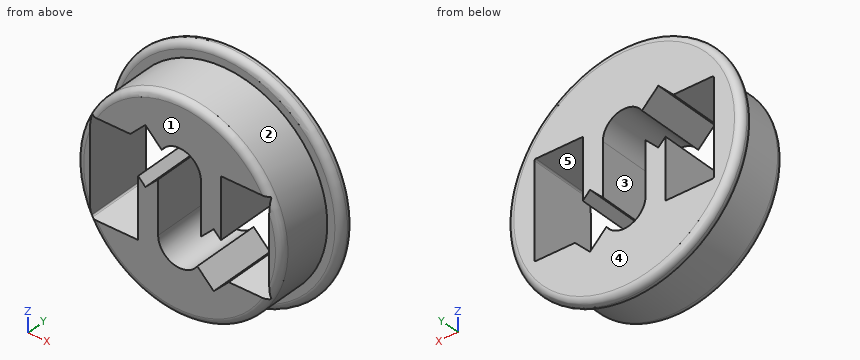
```python
from build123d import *

# Parameters (mm, degrees)
SKETCH1_R           = 7.45
BOSS_EXTRUDE1_DEPTH = 4
SKETCH2_R           = 8.5
BOSS_EXTRUDE2_DEPTH = 1
SKETCH3_W           = 3.5
SKETCH3_H           = 3.5
CUT_EXTRUDE1_DEPTH  = 14.019216566
CUT_EXTRUDE2_DEPTH  = 14.019216566
CUT_EXTRUDE3_DEPTH  = 14.019216566
FILLET3_R           = 0.5
FILLET5_R           = 0.1


with BuildPart() as part:
    # Sketch1 → Boss-Extrude1 (new body)
    with BuildSketch(Plane(origin=(0, 0, 0), x_dir=(1, 0, 0), z_dir=(0, 1, 0))):
        with Locations(Location((0, 0, 0), (0, 0, 270))):
            Circle(SKETCH1_R)
    extrude(amount=BOSS_EXTRUDE1_DEPTH)

    # Sketch2 → Boss-Extrude2 (add)
    with BuildSketch(Plane(origin=(0, 4, 0), x_dir=(1, 0, 0), z_dir=(0, 1, 0))):
        with Locations(Location((0, 0, 0), (0, 0, 270))):
            Circle(SKETCH2_R)
    extrude(amount=BOSS_EXTRUDE2_DEPTH)

    # Sketch3 → Cut-Extrude1 (cut, through all)
    with BuildSketch(Plane(origin=(0, 5, 0), x_dir=(1, 0, 0), z_dir=(0, 1, 0))):
        with Locations((-4.75, 1.75)):
            Rectangle(SKETCH3_W, SKETCH3_H)
        with Locations((-4.75, -1.75)):
            Rectangle(SKETCH3_W, SKETCH3_H)
        with Locations((4.75, -1.75)):
            Rectangle(SKETCH3_W, SKETCH3_H)
        with Locations((4.75, 1.75)):
            Rectangle(SKETCH3_W, SKETCH3_H)
    extrude(amount=-CUT_EXTRUDE1_DEPTH, mode=Mode.SUBTRACT)

    # Sketch3<4> → Cut-Extrude2 (cut, through all)
    with BuildSketch(Plane(origin=(0, 5, 0), x_dir=(1, 0, 0), z_dir=(0, 1, 0))):
        with BuildLine():
            Line((-1.55, -2.55), (-1.55, 2.55))
            ThreePointArc((-1.55, 2.55), (0, 4.1), (1.55, 2.55))
            Line((1.55, 2.55), (1.55, -2.55))
            ThreePointArc((1.55, -2.55), (0, -4.1), (-1.55, -2.55))
        make_face()
    extrude(amount=-CUT_EXTRUDE2_DEPTH, mode=Mode.SUBTRACT)

    # Sketch3<5> → Cut-Extrude3 (cut, through all)
    with BuildSketch(Plane(origin=(0, 5, 0), x_dir=(1, 0, 0), z_dir=(0, 1, 0))):
        Polygon((0.353553391, 2.474873734), (2.474873734, 4.596194078), (4.596194078, 2.474873734), (2.474873734, 0.353553391), align=None)
        Polygon((-4.596194078, -2.474873734), (-2.474873734, -4.596194078), (-0.353553391, -2.474873734), (-2.474873734, -0.353553391), align=None)
    extrude(amount=-CUT_EXTRUDE3_DEPTH, mode=Mode.SUBTRACT)

    # Fillet3
    # the kernel refuses this fillet: 0.5 mm, written as the material it takes off along each edge
    with BuildSketch(Plane(origin=(0, 0, 0), x_dir=(0, 0, 1), z_dir=(-1, 0, 0))) as fillet3_piece_1:
        with BuildLine():
            CenterArc((7.45 - FILLET3_R, FILLET3_R), FILLET3_R, 270, 90)
            Line((7.45 - FILLET3_R, 0), (7.45, 0))
            Line((7.45, 0), (7.45, FILLET3_R))
        make_face()
    revolve(axis=Axis((0, 0, 0), (0, 1, 0)), mode=Mode.SUBTRACT)
    with BuildSketch(Plane(origin=(0, 4, 0), x_dir=(0, 0, 1), z_dir=(-1, 0, 0))) as fillet3_piece_2:
        with BuildLine():
            CenterArc((8.5 - FILLET3_R, FILLET3_R), FILLET3_R, 270, 90)
            Line((8.5 - FILLET3_R, 0), (8.5, 0))
            Line((8.5, 0), (8.5, FILLET3_R))
        make_face()
    revolve(axis=Axis((0, 4, 0), (0, 1, 0)), mode=Mode.SUBTRACT)
    with BuildSketch(Plane(origin=(0, 5, 0), x_dir=(0, 0, 1), z_dir=(-1, 0, 0))) as fillet3_piece_3:
        with BuildLine():
            CenterArc((8.5 - FILLET3_R, -FILLET3_R), FILLET3_R, 0, 90)
            Line((8.5 - FILLET3_R, 0), (8.5, 0))
            Line((8.5, 0), (8.5, -FILLET3_R))
        make_face()
    revolve(axis=Axis((0, 5, 0), (0, 1, 0)), mode=Mode.SUBTRACT)

    # Fillet5
    fillet5_edges = [part.edges().sort_by_distance(p)[0] for p in [
        (-6.5, 2.62448081, 3.5),
        (-6.5, 2.62448081, -3.5),
        (6.5, 2.62448081, 3.5),
        (6.5, 2.62448081, -3.5),
    ]]
    fillet(fillet5_edges, radius=FILLET5_R)


solid = part.part
```
For this review, take the finished solid that the model builds, in its own axes (mm). Face numbers are marked on the shaded views. A direction names the side the tool comes from. Round coordinates to 2 decimals unless told otherwise and drop trailing zeros. Write each loop counter-clockwise with the first axis right and the second up, starting at its lowest first coordinate (ties: lowest second). Pieces come first, ordered by that corner, then holes.
1) Take a section at B-B on z = 0. Give the boundary of the cut face in (x, y).
Answer below:
outline: (-8, 4) - (-7.45, 4) - (-7.45, 0.5) arc R0.5 ccw to (-6.95, 0) - (-6.5, 0) - (-6.5, 5) - (-8, 5) arc R0.5 ccw to start; (-3, 0) - (-1.55, 0) - (-1.55, 5) - (-3, 5) - close; (1.55, 0) - (3, 0) - (3, 5) - (1.55, 5) - close; (6.5, 0) - (6.95, 0) arc R0.5 ccw to (7.45, 0.5) - (7.45, 4) - (8, 4) arc R0.5 ccw to (8, 5) - (6.5, 5) - close
2) Mouldability with a two-part tool opening along X and no side actions: class the marked faces 1, 2 and 3 as +X half, -X half, draft (parallel to the pull), parting line (faces both ways), or undercut.
Answer below:
face 1: draft
face 2: parting line
face 3: undercut
3) Take a section at C-C on y = 1.8. Give the boundary of the cut face in (x, z).
Answer below:
outline: circle Ø14.9 at (0, 0); hole (-6.5, -3.4) arc R0.1 ccw to (-6.4, -3.5) - (-3, -3.5) - (-3, 0.88) - (-2.47, 0.35) - (-1.55, 1.28) - (-1.55, -2.55) arc R1.55 ccw to (1.29, -3.41) - (2.47, -4.6) - (3.57, -3.5) - (6.4, -3.5) arc R0.1 ccw to (6.5, -3.4) - (6.5, 3.4) arc R0.1 ccw to (6.4, 3.5) - (3, 3.5) - (3, -0.88) - (2.47, -0.35) - (1.55, -1.28) - (1.55, 2.55) arc R1.55 ccw to (-1.29, 3.41) - (-2.47, 4.6) - (-3.57, 3.5) - (-6.4, 3.5) arc R0.1 ccw to (-6.5, 3.4) - close
4) Insertion check: pin 1 Ø1.5 at (y, z) = (1.5, -1) entering from -X; pin 2 Ø3 at (y, z) = (3.5, -1.5) entering from +X; pin 3 Ø2.5 at (x, y) = (5, 3) entering from +Z. Each pin has a flat end and moves straight along its axis. Give the tip position at first contact, or say it passes through.
Answer below:
pin 1: stops at x = -7.45
pin 2: stops at x = 8.49
pin 3: stops at z = 7.04
5) For line 1 along X through (y, z) = (2.65, 1.75); line 2 along X through (y, z) = (1.45, -1); line 3 along X through (y, z) = (2.7, 1), list the stretches that pass through material, from the lowest coordinate up.
Answer below:
line 1: x = -7.24 to -6.5, 1.55 to 3, 6.5 to 7.24
line 2: x = -7.38 to -6.5, -3 to -1.55, 1.55 to 1.83, 6.5 to 7.38
line 3: x = -7.38 to -6.5, -1.83 to -1.55, 1.55 to 3, 6.5 to 7.38
6) Take a section at A-A on x = 0. Give the boundary of the cut face in (y, z), then the cut area to 3 significant figures.
Answer below:
outline: (0, -6.95) arc R0.5 ccw to (0.5, -7.45) - (4, -7.45) - (4, -8) arc R0.5 ccw to (5, -8) - (5, -4.1) - (0, -4.1) - close; (0, 4.1) - (5, 4.1) - (5, 8) arc R0.5 ccw to (4, 8) - (4, 7.45) - (0.5, 7.45) arc R0.5 ccw to (0, 6.95) - close
area: 35.3 mm2
7) Machinability: for the marked faces 4 and 5, which of the approach directions +Z, -Z, +X, -X, +Y, -Y give a long, thin tool a straight path to every point of the face, cutting with its end or side? Answer none if there is none.
Answer below:
face 4: +Z, -Z, +X, -X, +Y
face 5: +Y, -Y
